Check sheet for the modelled part. Datum: model origin and axes. Units: mm. A direction names the side the tool comes from. Round coordinates to 2 decimals unless told otherwise and drop trailing zeros. Order: outer loops, then holes, each group sorted by start corner. A loop starts at its lowest first (then second) coordinate and runs counter-clockwise, first axis right, second up.
Q1. Cross-section at D-D on x = 15. Record the cut outline in (y, z).
Q2. Scan lines: probe 1 along Z at (x, y) = (8.5, -8); probe 2 along X at (y, z) = (-3, -52); probe 3 along X at (y, z) = (-13.5, -43). Record each from-to range of solid material in increasing order.
Q3. Cross-section at C-C on z = -38.5. Record the cut outline in (x, y), then the cut area to 3 significant figures.
Q4. Mould release check, pull along Z, two halves, no side actions. Record for faces 1 (the flat face through (19.712, -12.522, -3.188)), 2 (the flat face through (-23.667, -13, -49)), 3 (the flat face through (-2, -13, -55.732)), 4 (the flat face through (-20, -13, -27.942)): +Z half, -Z half, draft (parallel to the pull), parting line (faces both ways), or undercut.
Q5. Depth check by flat-ended pin: P1, Ø15, axis at x = 16, y = -18.5, coming from the +Z side; P2, Ø5, axis at x = -20.5, z = -30.5, coming from the +Y side; P3, Ø11.5, axis at x = -18.5, y = -17.5, coming from the +Z side (3 decimals); P4, Ø6.5, axis at y = -8.5, z = -50.5, coming from the +X side. Enter the tip coordinate at first touch or a pass-through.
Q6. Cross-section at B-B on y = -15.5. Record the cut outline in (x, z), then the cut area to 3 significant figures.
Q7. Cross-section at A-A on x = -21. Record the cut outline in (y, z), then the cut area to 3 significant figures.
Q8. Set-up check for faces 5 (the flat face through (-16, -13, -43.212)), 6 (the flat face through (20.613, -13, -50)), 7 (the flat face through (7.016, -13, -36)): record each of +Z, -Z, +X, -X, +Y, -Y from which the full face is reachable in a straight line by a thin tool's end or side.
from build123d import *

# Parameters (mm, degrees)
F0_W     = 16.2341720425
F0_H     = 15.2690820396
F1_DEPTH = 25.4
F2_DEPTH = 25.4


# Not quite as in the source:
# - a feature names something its author has since deleted; it is built from what else it names


with BuildPart() as f1:
    # F0 (on Front) → F1 (new body)
    with BuildSketch(Plane.XZ):
        Polygon((-9.2177884653, -27.9424227774), (7.0163835771, -27.9424227774), (27.7444086969, -27.9424227774), (27.7444086969, -9.1097736731), (11.4521000938, 2.9011261649), (-12.0625765994, 2.9011261649), (-29.7747123986, -9.1097736731), (-29.7747123986, -27.9424227774), align=None)
        with Locations((-1.1007024441, -35.5769637972)):
            Rectangle(F0_W, F0_H)
    extrude(amount=F1_DEPTH)

    # F0 (on Front) → F2 (join)
    with BuildSketch(Plane.XZ):
        Polygon((-23.6670821905, -55.7321608067), (20.6132540479, -55.7321608067), (20.6132540479, -43.211504817), (7.0163835771, -43.211504817), (-9.2177884653, -43.211504817), (-23.6670821905, -43.211504817), align=None)
    extrude(amount=F2_DEPTH)


solid = f1.part
Results found:
1. outline: (-25.4, -55.73) - (0, -55.73) - (0, -43.21) - (-25.4, -43.21) - close; (-25.4, -27.94) - (0, -27.94) - (0, 0.29) - (-25.4, 0.29) - close
2. probe 1: z = -55.73 to -43.21, -27.94 to 2.9
2. probe 2: x = -23.67 to 20.61
2. probe 3: x = -9.22 to 7.02
3. outline: (-9.22, -25.4) - (7.02, -25.4) - (7.02, 0) - (-9.22, 0) - close
3. area: 412 mm2
4. face 1: +Z half
4. face 2: draft
4. face 3: -Z half
4. face 4: undercut
5. P1: stops at z = 2.9
5. P2: passes through
5. P3: stops at z = 2.435
5. P4: stops at x = 20.61
6. outline: (-29.77, -27.94) - (-9.22, -27.94) - (-9.22, -43.21) - (-23.67, -43.21) - (-23.67, -55.73) - (20.61, -55.73) - (20.61, -43.21) - (7.02, -43.21) - (7.02, -27.94) - (27.74, -27.94) - (27.74, -9.11) - (11.45, 2.9) - (-12.06, 2.9) - (-29.77, -9.11) - close
6. area: 2,370 mm2
7. outline: (-25.4, -55.73) - (0, -55.73) - (0, -43.21) - (-25.4, -43.21) - close; (-25.4, -27.94) - (0, -27.94) - (0, -3.16) - (-25.4, -3.16) - close
7. area: 948 mm2
8. face 5: -X, +Y, -Y
8. face 6: -Z, +X, +Y, -Y
8. face 7: +X, +Y, -Y
